Solid Edge part; units mm, degrees
sketch "Sketch1" plane through (0, 0, 0) normal (0, -1, 0) x (1, 0, 0)
  line L0 (7.5, 0) -> (7.5, 10)
  line L1 (7.5, 10) -> (-7.5, 10)
  line L2 (-7.5, 10) -> (-7.5, 0)
  line L3 (-7.5, 0) -> (7.5, 0)
revolve "RevolvedProtrusion1" add sketch "Sketch1" angle 360 about axis through (-15, 0, 0) along (1, 0, 0)
sketch "Sketch2" plane through (7.5, 0, 0) normal (1, 0, 0) x (0, 1, 0)
  line L0 (-7, 7.1414) -> (-7, -7.1414)
  arc A0 (-7, -7.1414) -> (-7, 7.1414) centre (0, 0) cw
  line L1 (7, 7.1414) -> (7, -7.1414)
  arc A1 (7, 7.1414) -> (7, -7.1414) centre (0, 0) cw
extrude "VaciadoExtruido_1" cut sketch "Sketch2" against normal blind 7
hole "Agujero_1" at (-7.5, 0, 0) direction (1, 0, 0) diameter 8.376 end up to next start chamfer 1 start chamfer angle 45 end chamfer 1 end chamfer angle 45
CAD build for the part. Positions are in the model's coordinates, mm. A direction names the side the tool comes from. Coordinates: 2 decimals unless noted, no trailing zeros. Loops run counter-clockwise (first coordinate to the right, second up) from the corner with the lowest first, then second, coordinate; pieces in that order, holes last. Notation, with made-up numbers: (-29, 36) - (25, 36) arc R12 ccw to (25, 57) - close; hole circle Ø4 at (51, -12). An arc over 180 degrees is marked (long way). Use CSV: the item, a comma, the result in double quotes. Start each with the question number.
Q1. Two-plate mould, pull along Z, no slides. Class faces 4 (the cylindrical face through (-2, 0, -10)), 5 (the cylindrical face through (-0.091, 2.83, -3.087)), 6 (the flat face through (4, 7, 0)): +Z half, -Z half, draft (parallel to the pull), parting line (faces both ways), or undercut.
Q2. Cut at D-D, the plane z = -6. List the corners of the cut face in (x, y).
Q3. Probe probe 1 along Y at (x, z) = (-2, 0); probe 2 along Y at (x, z) = (2.25, 5). List the from-to ranges inside material, lowest first. Write a range as from..to.
Q4. Cut at B-B, the plane x = 5.25. List the corners of the cut face in (y, z).
Q5. Cut at A-A, the plane y = 0. List the corners of the cut face in (x, z).
Q6. Drop flat-ended pins along their axis: P1, Ø0.9, axis at y = -8.5, z = -2.5, coming from the +X side; P2, Ø3, axis at x = 4.5, y = -2, coming from the -Z side; P3, Ø2, axis at x = 3, z = -2, coming from the +Y side. Give the stop position or say it passes through.
Q7. Cut at C-C, the plane z = 0. List the corners of the cut face in (x, y).
Q8. 3-axis set-ups, long thin cutter, end or side, ignore diameter. For faces 1 (the flat face through (7.5, -5, 2)), 2 (the flat face through (4, -7, 0)), 3 (the flat face through (0.5, 8, 0)): which of +Z, -Z, +X, -X, +Y, -Y reach the whole face in a straight line?
Here are the results:
1,face 4,"parting line"
1,face 5,"undercut"
1,face 6,"draft"
2,outline,"(-7.5, -8) - (0.5, -8) - (0.5, -7) - (7.5, -7) - (7.5, 7) - (0.5, 7) - (0.5, 8) - (-7.5, 8) - close"
3,probe 1,"-10..-4.19, 4.19..10"
3,probe 2,"-7..7"
4,outline,"(-7, -7.14) arc R10 ccw to (7, -7.14) - (7, 7.14) arc R10 ccw to (-7, 7.14) - close; hole circle Ø8.38 at (0, 0)"
5,outline,"(-7.5, -10) - (7.5, -10) - (7.5, -5.19) - (6.5, -4.19) - (-6.5, -4.19) - (-7.5, -5.19) - close; (-7.5, 5.19) - (-6.5, 4.19) - (6.5, 4.19) - (7.5, 5.19) - (7.5, 10) - (-7.5, 10) - close"
6,P1,"x = 0.5"
6,P2,"z = -9.99"
6,P3,"y = 7"
7,outline,"(-7.5, -10) - (0.5, -10) - (0.5, -7) - (7.5, -7) - (7.5, -5.19) - (6.5, -4.19) - (-6.5, -4.19) - (-7.5, -5.19) - close; (-7.5, 5.19) - (-6.5, 4.19) - (6.5, 4.19) - (7.5, 5.19) - (7.5, 7) - (0.5, 7) - (0.5, 10) - (-7.5, 10) - close"
8,face 1,"+Z, -Z, +X, +Y, -Y"
8,face 2,"+Z, -Z, +X, -Y"
8,face 3,"+Z, -Z, +X, +Y"
